from build123d import *

# Parameters (mm, degrees)
F1_DEPTH = 3.175


# Not quite as in the source:
# - a feature names something its author has since deleted; it is built from what else it names


with BuildPart() as f1:
    # F0 (on Top) → F1 (new body)
    with BuildSketch(Plane.XY):
        Polygon((6.0392088785, 8.3122579143), (0, 6.35), (-6.0392088785, 8.3122579143), (-6.0392088785, 1.9622579143), (-9.7716452305, -3.175), (-3.7324363521, -5.1372579143), (0, -10.2745158286), (3.7324363521, -15.4117737428), (3.7324363521, -21.7617737428), (9.7716452305, -19.7995158286), (15.810854109, -21.7617737428), (15.810854109, -15.4117737428), (19.5432904611, -10.2745158286), (25.5824993395, -8.3122579143), (31.621708218, -10.2745158286), (31.621708218, -3.9245158286), (35.3541445701, 1.2127420857), (29.3149356916, 3.175), (25.5824993395, 8.3122579143), (21.8500629875, 13.4495158286), (21.8500629875, 19.7995158286), (15.810854109, 17.8372579143), (9.7716452305, 19.7995158286), (9.7716452305, 13.4495158286), align=None)
        Polygon((9.4541452305, -19.5688385759), (4.0499363521, -21.3247724831), (4.0499363521, -15.6424509955), (9.4541452305, -13.8865170883), align=None, mode=Mode.SUBTRACT)
        Polygon((0.5137257914, -10.4414354567), (5.9179346699, -8.6855015495), (9.2567076833, -13.2829899238), (3.8537105606, -15.0385301076), align=None, mode=Mode.SUBTRACT)
        Polygon((-9.2579194391, -3.0080803719), (-5.9179346699, 1.5890142791), (-0.5137257914, -0.1669196281), (-3.8537105606, -4.7640142791), align=None, mode=Mode.SUBTRACT)
        Polygon((-0.0007489063, -0.5411940443), (3.3399847692, -5.1372579143), (0, -9.7343525653), (-3.3399847692, -5.1372579143), align=None, mode=Mode.SUBTRACT)
        Polygon((3.9286621435, -5.4073395459), (8.9404194391, -3.7789208878), (5.842983087, -8.0421762826), (0.8312257914, -9.6705949407), align=None, mode=Mode.SUBTRACT)
        Polygon((9.7716452305, -3.7151632633), (13.1116299997, -8.3122579143), (9.7723941368, -12.9083217842), (6.4316604613, -8.3122579143), align=None, mode=Mode.SUBTRACT)
        Polygon((9.2579194391, -3.0080803719), (3.8537105606, -4.7640142791), (0.5149375472, -0.1665259048), (5.9179346699, 1.5890142791), align=None, mode=Mode.SUBTRACT)
        Polygon((10.0891452305, -2.9443227474), (10.0891452305, 2.7379987403), (15.493354109, 0.9820648331), (15.493354109, -4.7002566545), align=None, mode=Mode.SUBTRACT)
        Polygon((15.493354109, -15.6424509955), (15.493354109, -21.3247724831), (10.0891452305, -19.5688385759), (10.0891452305, -13.8865170883), align=None, mode=Mode.SUBTRACT)
        Polygon((13.6253557912, -8.6855015495), (19.0295646696, -10.4414354567), (15.6895799004, -15.0385301076), (10.285371022, -13.2825962005), align=None, mode=Mode.SUBTRACT)
        Polygon((15.6146283176, -5.4073395459), (18.7120646696, -9.6705949407), (13.700307374, -8.0421762826), (10.602871022, -3.7789208878), align=None, mode=Mode.SUBTRACT)
        Polygon((19.2257904611, -9.2973513055), (16.128354109, -5.0340959107), (16.128354109, 0.2355775627), (19.2257904611, -4.0276778321), align=None, mode=Mode.SUBTRACT)
        Polygon((19.8607904611, -9.8375145688), (19.8607904611, -4.1551930812), (25.2649993395, -2.399259174), (25.2649993395, -8.0815806616), align=None, mode=Mode.SUBTRACT)
        Polygon((31.304208218, -9.8375145688), (25.8999993395, -8.0815806616), (25.8999993395, -2.399259174), (31.304208218, -4.1551930812), align=None, mode=Mode.SUBTRACT)
        Polygon((-5.7217088785, 7.8752566545), (-0.3175, 6.1193227474), (-0.3175, 0.4370012597), (-5.7217088785, 2.1929351669), align=None, mode=Mode.SUBTRACT)
        Polygon((5.7217088785, 7.8752566545), (5.7217088785, 2.1929351669), (0.3175, 0.4370012597), (0.3175, 6.1193227474), align=None, mode=Mode.SUBTRACT)
        Polygon((6.3567088785, 2.0654199178), (6.3567088785, 7.3350933912), (9.4541452305, 3.0718379964), (9.4541452305, -2.1978354769), align=None, mode=Mode.SUBTRACT)
        Polygon((9.967871022, 3.4450816317), (6.8704346699, 7.7083370264), (11.8821919655, 6.0799183683), (14.9796283176, 1.8166629736), align=None, mode=Mode.SUBTRACT)
        Polygon((6.5529346699, 8.4791775424), (9.8929194391, 13.0762721934), (15.2971283176, 11.3203382862), (11.9571435484, 6.7232436352), align=None, mode=Mode.SUBTRACT)
        Polygon((25.0675617923, -1.7957320095), (19.6645646696, -3.5512721934), (16.3245799004, 1.0458224576), (21.7287887789, 2.8017563648), align=None, mode=Mode.SUBTRACT)
        Polygon((15.810854109, 1.752905349), (12.4708693398, 6.35), (15.8101052028, 10.94606387), (19.1508388782, 6.35), align=None, mode=Mode.SUBTRACT)
        Polygon((21.6538371961, 3.4450816317), (16.6420799004, 1.8166629736), (19.7395162525, 6.0799183683), (24.7512735481, 7.7083370264), align=None, mode=Mode.SUBTRACT)
        Polygon((25.5832482458, -1.42106387), (22.2425145703, 3.175), (25.5824993395, 7.772094651), (28.9224841087, 3.175), align=None, mode=Mode.SUBTRACT)
        Polygon((29.4362099002, 2.8017563648), (34.8404187786, 1.0458224576), (31.5004340094, -3.5512721934), (26.096225131, -1.7953382862), align=None, mode=Mode.SUBTRACT)
        Polygon((21.7287887789, 13.0762721934), (25.0687735481, 8.4791775424), (19.6645646696, 6.7232436352), (16.3257916562, 11.3207320095), align=None, mode=Mode.SUBTRACT)
        Polygon((10.0891452305, 13.6801930812), (10.0891452305, 19.3625145688), (15.493354109, 17.6065806616), (15.493354109, 11.924259174), align=None, mode=Mode.SUBTRACT)
        Polygon((16.128354109, 17.6065806616), (21.5325629875, 19.3625145688), (21.5325629875, 13.6801930812), (16.128354109, 11.924259174), align=None, mode=Mode.SUBTRACT)
    extrude(amount=F1_DEPTH)


solid = f1.part
The model under review builds one solid part; all positions refer to its coordinate system, in mm. A direction names the side the tool comes from. Coordinates: 2 decimals unless noted, no trailing zeros. Loops run counter-clockwise (first coordinate to the right, second up) from the corner with the lowest first, then second, coordinate; pieces in that order, holes last.
(1) Consider section A-A, the plane y = 17. Give the boundary of the cut face in (x, z) (3 decimals).
Determined:
outline: (9.772, 0) - (10.089, 0) - (10.089, 3.175) - (9.772, 3.175) - close; (15.493, 0) - (16.128, 0) - (16.128, 3.175) - (15.493, 3.175) - close; (21.533, 0) - (21.85, 0) - (21.85, 3.175) - (21.533, 3.175) - close
(2) Consider section C-C, the plane z = 2.3. Give the number of separate pieces and of enclosed holes in the cut face, plus the area to 3 significant figures.
Determined:
separate pieces: 1
enclosed holes: 27
area: 205 mm2
(3) Draft analysis for pull direction Y (two halves, no side actions). For faces 1 (the flat face through (25.265, -5, 2)), 2 (the flat face through (-2.98, 7.32, 1.57)), 3 (the flat face through (31.622, -7, 2)), state which applies: +Y half, -Y half, draft (parallel to the pull), parting line (faces both ways), or undercut.
Determined:
face 1: undercut
face 2: +Y half
face 3: draft
(4) Tool access review of faces 4 (the flat face through (-7.9, -0.6, 1.6)), 5 (the flat face through (22.521, -9.307, 1.565)), 6 (the flat face through (3.178, -9.576, 1.565)): name each direction out of +Z, -Z, +X, -X, +Y, -Y from which nothing blocks a thin tool from reaching the whole face with its end or side.
Determined:
face 4: +Z, -Z, -X, +Y
face 5: +Z, -Z, -Y
face 6: +Z, -Z
(5) Wall thickness on L1, parallel to X at y = -16, z = 1.8; L2, parallel to X at y = 16, z = 1.8; L3, parallel to Y at x = 31, z = 1.35: over which ranges is each line inside the solid? List them lowest first.
Determined:
L1: x = 3.73 to 4.05, 9.45 to 10.09, 15.49 to 15.81
L2: x = 9.77 to 10.09, 15.49 to 16.13, 21.53 to 21.85
L3: y = -10.07 to -9.74, -4.06 to -3.39, 2.29 to 2.63
(6) Insertion check: P1, Ø1.6, axis at y = 17, z = 1.5, coming from the -X side; P2, Ø1, axis at x = 20.5, z = 2, coming from the +Y side; P3, Ø1.6, axis at y = 5, z = 2, coming from the +X side. Each pin has a flat end and moves straight along its axis. Give the tip position at first contact, or say it passes through.
Determined:
P1: stops at x = 9.77
P2: stops at y = 19.52
P3: stops at x = 28.57
(7) Consider section B-B, the plane x = -7. Give the boundary of the cut face in (y, z) (3 decimals).
Determined:
outline: (-4.076, 0) - (-3.742, 0) - (-3.742, 3.175) - (-4.076, 3.175) - close; (0.1, 0) - (0.64, 0) - (0.64, 3.175) - (0.1, 3.175) - close
